Source: CAD feature listing. Evaluate the final solid. Frame: model axes, mm. A direction names the side the tool comes from. Round coordinates to 2 decimals unless told otherwise and drop trailing zeros. Order: outer loops, then holes, each group sorted by start corner. A loop starts at its lowest first (then second) coordinate and runs counter-clockwise, first axis right, second up. Notation, with made-up numbers: (32, 25.5) - (53, 25.5) arc R29 ccw to (53, 58.5) - close; hole circle Ø10 at (71.25, 70.25). An arc over 180 degrees is marked (long way). Return JSON: item names as keys, results as strings. Group by question number.
1) Section C-C, the plane x = 0.75. Return loops of the section in (y, z).
2) Access query for faces 5 (the cylindrical face through (0.54, -2.44, -3.94)), 6 (the flat face through (0, -3, 50)). Directions: +Z, -Z, +X, -X, +Y, -Y. A direction counts if a zero-diameter tool reaches every point of the face in a straight line with its end or side. Return the directions, or none.
3) Ray query, line 1 (Y direction, x = 0, z = 47.45); line 2 (Z direction, x = -2.25, y = -1); line 3 (Z direction, x = 3.25, y = 1). Return the intervals inside material, ascending. Write a range as from..to.
4) Mould query, pull axis X, two halves, no side actions, for faces 1 (the flat face through (3.5, 0, 25)), 2 (the flat face through (0, 0, -8)), 3 (the flat face through (-3.5, 0, 25)), 4 (the flat face through (0, 0, 10)). Classes: pulls with the +X half, pulls with the -X half, needs draft (parallel to the pull), parting line crosses it, or undercut.
5) Section A-A, the plane y = -1.5. Return loops of the section in (x, z), plus the area to 3 significant figures.
6) Section D-D, the plane z = 3. Return loops of the section in (x, y), plus the area to 3 significant figures.
7) Contact query for a flat-ended pin moving along its axis: P1, Ø2.5, axis at x = 0, y = 1, coming from the +Z side. Output: stop coordinate, or through.
8) Section B-B, the plane z = 30. Return loops of the section in (x, y).
```python
from build123d import *

# Parameters (mm, degrees)
EXTRUDE_1_DEPTH     = 60
SKETCH_2_R          = 2.5
EXTRUDE_2_DEPTH     = 8
SKETCH_3_R          = 2.5
CUT_EXTRUDE_1_DEPTH = 50
SKETCH_4_R          = 11.437088518
CUT_EXTRUDE_2_DEPTH = 20
EXTRUDE_3_DEPTH     = 5
SKETCH_6_R          = 2.5
CUT_EXTRUDE_3_DEPTH = 16
EXTRUDE_5_DEPTH     = 5
SKETCH_9_R          = 2.5
CUT_EXTRUDE_4_DEPTH = 5


with BuildPart() as part:
    # 草图1 → 凸台-拉伸1 (new body)
    with BuildSketch(Plane.XY):
        Polygon((3.5, -2.020725942), (3.5, 2.020725942), (0, 4.041451884), (-3.5, 2.020725942), (-3.5, -2.020725942), (0, -4.041451884), align=None)
    extrude(amount=EXTRUDE_1_DEPTH)

    # 草图2 → 凸台-拉伸2 (add)
    with BuildSketch(Plane(origin=(0, 0, 0), x_dir=(-1, 0, 0), z_dir=(0, 0, -1))):
        Circle(SKETCH_2_R)
    extrude(amount=EXTRUDE_2_DEPTH)

    # 草图3 → 切除-拉伸1 (cut)
    with BuildSketch(Plane.XY.offset(60)):
        with Locations(Location((0, 0, 0), (0, 0, 180))):
            Circle(SKETCH_3_R)
    extrude(amount=-CUT_EXTRUDE_1_DEPTH, mode=Mode.SUBTRACT)

    # 草图4 → 切除-拉伸2 (cut)
    with BuildSketch(Plane.XY.offset(60)):
        with Locations((-0.3770193, 0.287149771)):
            Circle(SKETCH_4_R)
    extrude(amount=-CUT_EXTRUDE_2_DEPTH, mode=Mode.SUBTRACT)

    # 草图5 → 凸台-拉伸3 (add)
    with BuildSketch(Plane.XY.offset(40)):
        Polygon((0, 4.041451884), (-3.5, 2.020725942), (-3.5, -2.020725942), (0, -4.041451884), (3.5, -2.020725942), (3.5, 2.020725942), align=None)
    extrude(amount=EXTRUDE_3_DEPTH)

    # 草图6 → 切除-拉伸3 (cut)
    with BuildSketch(Plane.XY.offset(45)):
        Circle(SKETCH_6_R)
    extrude(amount=-CUT_EXTRUDE_3_DEPTH, mode=Mode.SUBTRACT)

    # 草图7 → 凸台-拉伸5 (add)
    with BuildSketch(Plane.XY.offset(45)):
        Polygon((-3.5, 2.020725942), (0, 4.041451884), (3.5, 2.020725942), (3.5, -2.020725942), (0, -4.041451884), (-3.5, -2.020725942), align=None)
    extrude(amount=EXTRUDE_5_DEPTH)

    # 草图9 → 切除-拉伸4 (cut)
    with BuildSketch(Plane.XY.offset(50)):
        with Locations(Location((0, 0, 0), (0, 0, 180))):
            Circle(SKETCH_9_R)
    extrude(amount=-CUT_EXTRUDE_4_DEPTH, mode=Mode.SUBTRACT)


solid = part.part
```
Geometry check:
{
 "1": {"outline": "(-3.61, 0) - (-2.38, 0) - (-2.38, -8) - (2.38, -8) - (2.38, 0) - (3.61, 0) - (3.61, 50) - (2.38, 50) - (2.38, 10) - (-2.38, 10) - (-2.38, 50) - (-3.61, 50) - close"},
 "2": {"face 5": "-Z", "face 6": "+Z, +X, -X, +Y, -Y"},
 "3": {"line 1": "-4.04..-2.5, 2.5..4.04", "line 2": "-8..10", "line 3": "0..50"},
 "4": {"face 1": "pulls with the +X half", "face 2": "needs draft", "face 3": "pulls with the -X half", "face 4": "undercut"},
 "5": {"outline": "(-3.5, 0) - (-2, 0) - (-2, -8) - (2, -8) - (2, 0) - (3.5, 0) - (3.5, 50) - (2, 50) - (2, 10) - (-2, 10) - (-2, 50) - (-3.5, 50) - close", "area": "222 mm2"},
 "6": {"outline": "(-3.5, -2.02) - (0, -4.04) - (3.5, -2.02) - (3.5, 2.02) - (0, 4.04) - (-3.5, 2.02) - close", "area": "42.4 mm2"},
 "7": {"P1": "z = 10"},
 "8": {"outline": "(-3.5, -2.02) - (0, -4.04) - (3.5, -2.02) - (3.5, 2.02) - (0, 4.04) - (-3.5, 2.02) - close; hole circle Ø5 at (0, 0)"}
}
